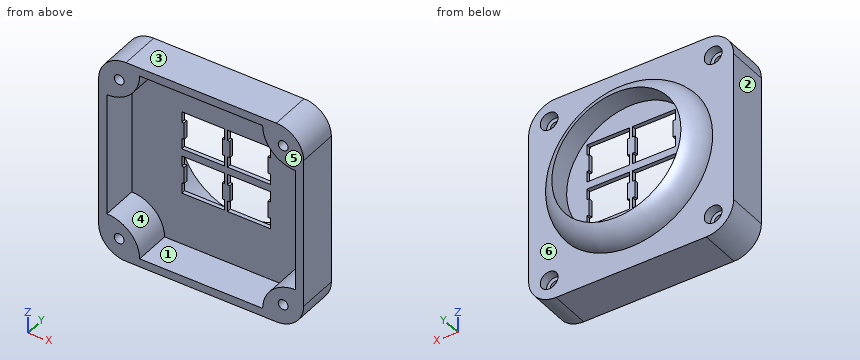
```python
from build123d import *

# Parameters (mm, degrees)
SKIZZE1_R                                            = 1.6
AUFSATZ_LINEAR_AUSTRAGEN1_DEPTH                      = 15
AUFSATZ_LINEAR_AUSTRAGEN2_DEPTH                      = 1.5
VERRUNDUNG1_R                                        = 10
VERRUNDUNG2_R                                        = 12
STIRNSENKUNG_F_R_M3_ZYLINDERSCHRAUBE_MIT_D           = 3.6
STIRNSENKUNG_F_R_M3_ZYLINDERSCHRAUBE_MIT_CBORE_D     = 6.5
STIRNSENKUNG_F_R_M3_ZYLINDERSCHRAUBE_MIT_CBORE_DEPTH = 3.4


with BuildPart() as part:
    # Skizze1 → Aufsatz-Linear austragen1 (new body)
    with BuildSketch(Plane(origin=(0, 0, 0), x_dir=(1, 0, 0), z_dir=(0, 1, 0))):
        Polygon((-37.5, 22.5), (-37.5, -37.5), (37.5, -37.5), (37.5, 37.5), (-35, 37.5), (-37.5, 37.5), align=None)
        with Locations(Location((-30, -30, 0), (0, 0, 270))):
            Circle(SKIZZE1_R, mode=Mode.SUBTRACT)
        with Locations(Location((30, -30, 0), (0, 0, 270))):
            Circle(SKIZZE1_R, mode=Mode.SUBTRACT)
        with Locations(Location((-30, 30, 0), (0, 0, 270))):
            Circle(SKIZZE1_R, mode=Mode.SUBTRACT)
        Polygon((-22.5, 22.5), (-22.5, 34.5), (22.5, 34.5), (22.5, 22.5), (34.5, 22.5), (34.5, -22.5), (22.5, -22.5), (22.5, -34.5), (-22.5, -34.5), (-22.5, -22.5), (-34.5, -22.5), (-34.5, 22.5), align=None, mode=Mode.SUBTRACT)
        with Locations(Location((30, 30, 0), (0, 0, 270))):
            Circle(SKIZZE1_R, mode=Mode.SUBTRACT)
    extrude(amount=-AUFSATZ_LINEAR_AUSTRAGEN1_DEPTH)

    # Skizze1<3> → Aufsatz-Linear austragen2 (add)
    with BuildSketch(Plane(origin=(0, 0, 0), x_dir=(1, 0, 0), z_dir=(0, 1, 0))):
        Polygon((22.5, 34.5), (-22.5, 34.5), (-22.5, 22.5), (-34.5, 22.5), (-34.5, -22.5), (-22.5, -22.5), (-22.5, -34.5), (22.5, -34.5), (22.5, -22.5), (34.5, -22.5), (34.5, 22.5), (22.5, 22.5), align=None)
        Polygon((-0.51468496, -5.28988496), (-1.35288496, -5.28988496), (-1.35288496, -11.41128496), (-0.51468496, -11.41128496), (-0.51468496, -15.34828496), (-1.35288496, -15.34828496), (-15.34828496, -15.34828496), (-16.18648496, -15.34828496), (-16.18648496, -11.41128496), (-15.34828496, -11.41128496), (-15.34828496, -5.28988496), (-16.18648496, -5.28988496), (-16.18648496, -1.35288496), (-15.34828496, -1.35288496), (-1.35288496, -1.35288496), (-0.51468496, -1.35288496), align=None, mode=Mode.SUBTRACT)
        Polygon((15.34828496, -15.34828496), (1.35288496, -15.34828496), (0.51468496, -15.34828496), (0.51468496, -11.41128496), (1.35288496, -11.41128496), (1.35288496, -5.28988496), (0.51468496, -5.28988496), (0.51468496, -1.35288496), (1.35288496, -1.35288496), (15.34828496, -1.35288496), (16.18648496, -1.35288496), (16.18648496, -5.28988496), (15.34828496, -5.28988496), (15.34828496, -11.41128496), (16.18648496, -11.41128496), (16.18648496, -15.34828496), align=None, mode=Mode.SUBTRACT)
        Polygon((-15.34828496, 15.34828496), (-1.35288496, 15.34828496), (-0.51468496, 15.34828496), (-0.51468496, 11.41128496), (-1.35288496, 11.41128496), (-1.35288496, 5.28988496), (-0.51468496, 5.28988496), (-0.51468496, 1.35288496), (-1.35288496, 1.35288496), (-15.34828496, 1.35288496), (-16.18648496, 1.35288496), (-16.18648496, 5.28988496), (-15.34828496, 5.28988496), (-15.34828496, 11.41128496), (-16.18648496, 11.41128496), (-16.18648496, 15.34828496), align=None, mode=Mode.SUBTRACT)
        Polygon((0.51468496, 5.28988496), (1.35288496, 5.28988496), (1.35288496, 11.41128496), (0.51468496, 11.41128496), (0.51468496, 15.34828496), (1.35288496, 15.34828496), (15.34828496, 15.34828496), (16.18648496, 15.34828496), (16.18648496, 11.41128496), (15.34828496, 11.41128496), (15.34828496, 5.28988496), (16.18648496, 5.28988496), (16.18648496, 1.35288496), (15.34828496, 1.35288496), (1.35288496, 1.35288496), (0.51468496, 1.35288496), align=None, mode=Mode.SUBTRACT)
    extrude(amount=-AUFSATZ_LINEAR_AUSTRAGEN2_DEPTH)

    # Verrundung1
    verrundung1_edges = [part.edges().sort_by_distance(p)[0] for p in [
        (37.5, -7.5, -37.5),
        (37.5, -7.5, 37.5),
        (-37.5, -7.5, 37.5),
        (-37.5, -7.5, -37.5),
    ]]
    fillet(verrundung1_edges, radius=VERRUNDUNG1_R)

    # Verrundung2
    verrundung2_edges = [part.edges().sort_by_distance(p)[0] for p in [
        (22.5, -8.25, 22.5),
        (-22.5, -8.25, 22.5),
        (22.5, -8.25, -22.5),
        (-22.5, -8.25, -22.5),
    ]]
    fillet(verrundung2_edges, radius=VERRUNDUNG2_R - 0.0001)  # a hair under: the kernel refuses the full size

    # Skizze3 → Rotation1 (revolve)
    with BuildSketch(Plane(origin=(0, 0, 0), x_dir=(0, 0, -1), z_dir=(1, 0, 0))):
        with BuildLine():
            Line((23.608930659, 0), (29.803663871, 0))
            ThreePointArc((29.803663871, 0), (27.936560085, 4.952643744), (23.608930659, 8))
            Line((23.608930659, 8), (23.608930659, 0))
        make_face()
    revolve(axis=Axis((0, 0, 0), (0, 1, 0)))

    # Stirnsenkung für M3 Zylinderschraube mit Innensechskant1 (through all)
    with Locations(Plane(origin=(0, 0, 0), x_dir=(1, 0, 0), z_dir=(0, 1, 0))):
        with Locations((-30, 30), (30, 30), (-30, -30), (30, -30)):
            CounterBoreHole(STIRNSENKUNG_F_R_M3_ZYLINDERSCHRAUBE_MIT_D / 2, STIRNSENKUNG_F_R_M3_ZYLINDERSCHRAUBE_MIT_CBORE_D / 2, STIRNSENKUNG_F_R_M3_ZYLINDERSCHRAUBE_MIT_CBORE_DEPTH)


solid = part.part
```
Can you work these out from the model? Positions are in its coordinate system, mm. Face numbers are marked on the shaded views. A direction names the side the tool comes from. Round coordinates to 2 decimals unless told otherwise and drop trailing zeros. Loops run counter-clockwise (first coordinate to the right, second up) from the corner with the lowest first, then second, coordinate; pieces in that order, holes last. Notation, with made-up numbers: (60, 70) -> (89, 70) arc R26 cw to (89, 105) -> close; hole circle Ø7 at (-31, -11). An arc over 180 degrees is marked (long way). One line per item, written item: value. Start each with the question number.
1. If we section it at B-B, the plane z = 0: Write out the boundary of the cut face in (x, y).
2. For pin 1 (23.5 mm diameter, centred on x = 9.5, z = -4, fed in from +Y); pin 2 (4 mm diameter, centred on x = -27.5, z = -9.5, fed in from +Y) (3 decimals); pin 3 (6 mm diameter, centred on x = 14, z = -22, fed in from -Y); pin 4 (2 mm diameter, centred on x = -30, z = 30, fed in from +Y), each with a flat end and sliding along its axis, tell me the tip position at first contact or that it passes through.
3. If we mould it in two halves opening along Z, with no side actions, what happens to the marked faces 1, 2 and 3? For each: pulls with the +Z half, pulls with the -Z half, needs draft (parallel to the pull), parting line crosses it, or undercut.
4. If we section it at A-A, the plane y = -6.75: Give the number of separate pieces and of enclosed holes in the cut face, then the cut area to 3 significant figures.
5. If I drill on probe 1 along X at (y, z) = (-1.4, 30); probe 2 along Z at (x, y) = (-30, -1.8), over which ranges is the centre line in solid material (lowest first)?
6. For the marked faces 4, 5 and 6, which set-ups out of +Z, -Z, +X, -X, +Y, -Y let a thin tool reach every point of the face, with its end or its side?
Calculated:
1. outline: (-37.5, -15) -> (-34.5, -15) -> (-34.5, -1.5) -> (34.5, -1.5) -> (34.5, -15) -> (37.5, -15) -> (37.5, 0) -> (29.8, 0) arc R9 ccw to (23.61, 8) -> (23.61, 0) -> (-23.61, 0) -> (-23.61, 8) arc R9 ccw to (-29.8, 0) -> (-37.5, 0) -> close
2. pin 1: stops at y = 0
2. pin 2: stops at y = 5.895
2. pin 3: stops at y = -1.5
2. pin 4: passes through
3. face 1: undercut
3. face 2: needs draft
3. face 3: pulls with the +Z half
4. separate pieces: 1
4. enclosed holes: 5
4. area: 1,190 mm²
5. probe 1: x = -37.18 to -33.25, -26.75 to 26.75, 33.25 to 37.18
5. probe 2: z = -37.18 to -33.25, -26.75 to -23.38, 23.38 to 26.75, 33.25 to 37.18
6. face 4: -Y
6. face 5: +Z, -Z, +X, -X, -Y
6. face 6: +Y
